Work out the finished part from the listing and answer in its coordinate system (mm). Face numbers are marked on the shaded views. A direction names the side the tool comes from. Round coordinates to 2 decimals unless told otherwise and drop trailing zeros. Write each loop counter-clockwise with the first axis right and the second up, starting at its lowest first coordinate (ties: lowest second). Pieces come first, ordered by that corner, then holes.
1. Straight lines are drawn through the part: probe 1 along X at (y, z) = (2.5, -32); probe 2 along Z at (x, y) = (20.5, 2.5); probe 3 along Z at (x, y) = (6, 9.5). For each, find the intervals that lie inside material, in ascending order.
2. Find section A-A (y = 6). Write down the section's boundary in (x, z).
3. Find section B-B (x = 3). Write down the section's boundary in (y, z), and give its area (3 significant figures).
4. Determine the mould class of the marked faces 3, 4 and 5 for opening direction X: pulls with the +X half, pulls with the -X half, needs draft (parallel to the pull), parting line crosses it, or undercut.
5. A flat-ended cylindrical pin translates along its axis: pin 1 Ø4 at (x, z) = (36.5, 10.5) entering from -Y. Find the tip coordinate at first contact, or state that the pin passes through.
6. Find section C-C (z = -17.5). Write down the section's boundary in (x, y), and give its area (3 significant figures).
7. A tool of negligible diameter and unlimited length cuts with its end or side. For the marked faces 1 and 2, from which of +Z, -Z, +X, -X, +Y, -Y can it reach the whole face along a straight path? Write none if from no direction.
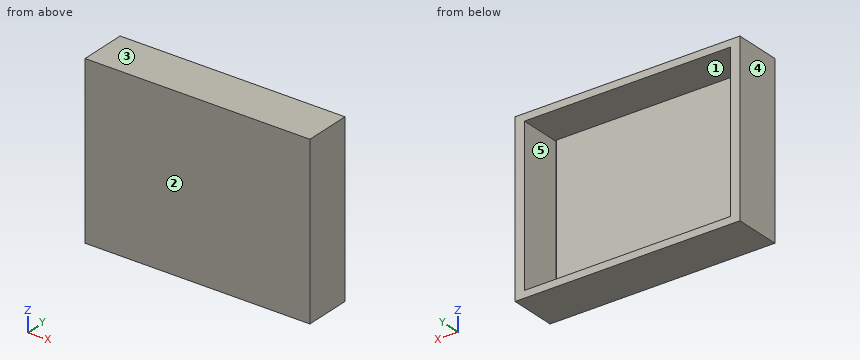
```python
from build123d import *

# Parameters (mm, degrees)
SKETCH_1_W          = 80
SKETCH_1_H          = 60
EXTRUDE_1_DEPTH     = 5
SKETCH_2_W          = 96
SKETCH_2_H          = 72
EXTRUDE_2_DEPTH     = 20
SKETCH_3_W          = 88
SKETCH_3_H          = 66
CUT_EXTRUDE_1_DEPTH = 18
SKETCH_5_W          = 80
SKETCH_5_H          = 60
EXTRUDE_3_DEPTH     = 5


with BuildPart() as part:
    # 草图1 → 凸台-拉伸1 (new body)
    with BuildSketch(Plane(origin=(0, 0, 0), x_dir=(1, 0, 0), z_dir=(0, 1, 0))):
        with Locations((5.833333333, 4.444444444)):
            Rectangle(SKETCH_1_W, SKETCH_1_H)
    extrude(amount=EXTRUDE_1_DEPTH)

    # 草图2 → 凸台-拉伸2 (add)
    with BuildSketch(Plane.XZ):
        with Locations((5.833333333, -2.444444444)):
            Rectangle(SKETCH_2_W, SKETCH_2_H)
    extrude(amount=-EXTRUDE_2_DEPTH)

    # 草图3 → 切除-拉伸1 (cut)
    with BuildSketch(Plane(origin=(0, 20, 0), x_dir=(1, 0, 0), z_dir=(0, 1, 0))):
        with Locations((5.833333333, 2.444444444)):
            Rectangle(SKETCH_3_W, SKETCH_3_H)
    extrude(amount=-CUT_EXTRUDE_1_DEPTH, mode=Mode.SUBTRACT)

    # 草图5 → 凸台-拉伸3 (add)
    with BuildSketch(Plane(origin=(0, 2, 0), x_dir=(1, 0, 0), z_dir=(0, 1, 0))):
        with Locations((5.833333333, 2.444444444)):
            Rectangle(SKETCH_5_W, SKETCH_5_H)
    extrude(amount=EXTRUDE_3_DEPTH)


solid = part.part
```
Worked answers:
1. probe 1: x = -42.17 to -38.17, -34.17 to 45.83, 49.83 to 53.83
1. probe 2: z = -38.44 to -35.44, -32.44 to 27.56, 30.56 to 33.56
1. probe 3: z = -38.44 to -35.44, 30.56 to 33.56
2. outline: (-42.17, -38.44) - (53.83, -38.44) - (53.83, 33.56) - (-42.17, 33.56) - close; (-34.17, -32.44) - (45.83, -32.44) - (45.83, 27.56) - (-34.17, 27.56) - close; hole (-38.17, -35.44) - (49.83, -35.44) - (49.83, 30.56) - (-38.17, 30.56) - close
3. outline: (0, -38.44) - (20, -38.44) - (20, -35.44) - (2, -35.44) - (2, -32.44) - (7, -32.44) - (7, 27.56) - (2, 27.56) - (2, 30.56) - (20, 30.56) - (20, 33.56) - (0, 33.56) - close
3. area: 552 mm2
4. face 3: needs draft
4. face 4: pulls with the -X half
4. face 5: undercut
5. pin 1: stops at y = 0
6. outline: (-42.17, 0) - (53.83, 0) - (53.83, 20) - (49.83, 20) - (49.83, 2) - (45.83, 2) - (45.83, 7) - (-34.17, 7) - (-34.17, 2) - (-38.17, 2) - (-38.17, 20) - (-42.17, 20) - close
6. area: 736 mm2
7. face 1: +Y
7. face 2: +Z, -Z, +X, -X, -Y
